The listing builds one solid part. Answer for the finished solid, in the listing's coordinates (mm). A direction names the side the tool comes from. Give positions to 0.01 mm unless a question says otherwise; leave off trailing zeros. Write each loop counter-clockwise with the first axis right and the second up, starting at its lowest first coordinate (ties: lowest second). Pieces come first, ordered by that corner, then holes. Notation, with made-up numbers: (60.5, 1) - (91.5, 1) arc R16 ccw to (91.5, 21) - close; hole circle Ø9 at (61.5, 62). An arc over 180 degrees is marked (long way). Answer as CSV lines item,"result". Start each with the question number.
(1) Find section A-A (x = 0). Write down the section's boundary in (y, z), then the cut area to 3 significant figures.
(2) Find section B-B (z = 9). Write down the section's boundary in (x, y), then the cut area to 3 significant figures.
(3) For faces 1 (the face through (15.294, 0, 5)), 2 (the face through (-9.228, -3.186, 2.465)), 3 (the face through (0, -4.7, 8)), determine the directions among +Z, -Z, +X, -X, +Y, -Y from which every point of the face is accessible in a straight line to the end or side of a thin tool.
(4) Find section C-C (z = 3.5). State how many separate pieces and enclosed holes the cut face has, then the cut area to 3 significant figures.
(5) Each of these flat-tipped pins is pushed along its axis until it touches: pin 1 Ø7 at (x, y) = (1.5, 2) entering from -Z; pin 2 Ø3 at (x, y) = (-11, -1.5) entering from -Z. Where does it stop, or does it pass through?
(6) Find section D-D (x = -7). Write down the section's boundary in (y, z), then the cut area to 3 significant figures.
(7) For a pull along X with two mould halves and no side action, classify faces 4 (the face through (0, -8, 0)), 5 (the face through (5.15, -1.77, 7.98)), 6 (the face through (-14.09, 7.44, 4.82)), 7 (the face through (14.154, -7.374, 4.816)) as pulls with the +X half, pulls with the -X half, needs draft (parallel to the pull), parting line crosses it, or undercut.
(8) Straight lines are drawn through the part: probe 1 along Y at (x, z) = (3, 1.5); probe 2 along X at (y, z) = (-1.5, 8.5); probe 3 along X at (y, z) = (4.25, 5.25). For each, find the intervals that lie inside material, in ascending order.
from build123d import *

# Parameters (mm, degrees)
SKETCH041_W     = 30.588764
SKETCH041_H     = 17.153068
PAD012_DEPTH    = 10
SKETCH042_W     = 18
SKETCH042_H     = 14
POCKET033_DEPTH = 6
POCKET034_DEPTH = 5
POCKET035_DEPTH = 10.001
SKETCH045_R     = 1.272634
PAD013_DEPTH    = 3
CHAMFER011_SIZE = 1
FILLET033_R     = 0.8
FILLET034_R     = 4
FILLET035_R     = 0.5


with BuildPart() as part:
    # Sketch041 → Pad012 (new body)
    with BuildSketch(Plane.XY):
        Rectangle(SKETCH041_W, SKETCH041_H)
    extrude(amount=PAD012_DEPTH)

    # Sketch042 → Pocket033 (cut)
    with BuildSketch(Plane.XY):
        Rectangle(SKETCH042_W, SKETCH042_H)
    extrude(amount=POCKET033_DEPTH, mode=Mode.SUBTRACT)

    # Sketch043 → Pocket034 (cut)
    with BuildSketch(Plane.XY):
        with BuildLine():
            ThreePointArc((-9.861316, 2.945018), (-12.806334, 0), (-9.861316, -2.945018))
            Line((-9.861316, -2.945018), (9.861316, -2.945018))
            ThreePointArc((9.861316, -2.945018), (12.806334, 0), (9.861316, 2.945018))
            Line((9.861316, 2.945018), (-9.861316, 2.945018))
        make_face()
    extrude(amount=POCKET034_DEPTH, mode=Mode.SUBTRACT)

    # Sketch044 → Pocket035 (cut, through all)
    with BuildSketch(Plane.XY):
        with BuildLine():
            ThreePointArc((-2.15, 1.3), (-5.15, -1.7), (-2.15, -4.7))
            Line((-2.15, -4.7), (2.15, -4.7))
            ThreePointArc((2.15, -4.7), (5.15, -1.7), (2.15, 1.3))
            Line((2.15, 1.3), (-2.15, 1.3))
        make_face()
    extrude(amount=POCKET035_DEPTH, mode=Mode.SUBTRACT)

    # Sketch045 (on Face21 of Pocket035) → Pad013 (join)
    with BuildSketch(Plane(origin=(0, 0, 6), x_dir=(1, 0, 0), z_dir=(0, 0, -1))):
        with Locations((-9.839489, 0)):
            Circle(SKETCH045_R)
        with Locations((9.839489, 0)):
            Circle(SKETCH045_R)
    extrude(amount=PAD013_DEPTH)

    # Chamfer011
    chamfer011_edges = [part.edges().sort_by_distance(p)[0] for p in [
        (8.566855, 0, 3),
        (-11.112123, 0, 3),
    ]]
    chamfer(chamfer011_edges, length=CHAMFER011_SIZE)

    # Fillet033
    fillet033_edges = [part.edges().sort_by_distance(p)[0] for p in [
        (9, 2.945018, 2.5),
        (9, -2.945018, 2.5),
        (9, 7, 3),
        (-9, 2.945018, 2.5),
        (-9, -2.945018, 2.5),
        (-9, -7, 3),
        (9, -7, 3),
        (-9, 7, 3),
    ]]
    fillet(fillet033_edges, radius=FILLET033_R)

    # Fillet034
    fillet034_edges = [part.edges().sort_by_distance(p)[0] for p in [
        (-15.294382, -8.576534, 5),
        (-15.294382, 8.576534, 5),
        (15.294382, 8.576534, 5),
        (15.294382, -8.576534, 5),
    ]]
    fillet(fillet034_edges, radius=FILLET034_R)

    # Fillet035
    fillet035_edges = [part.edges().sort_by_distance(p)[0] for p in [
        (0, 8.576534, 10),
        (-14.12281, 7.404962, 10),
        (14.12281, 7.404962, 10),
        (-15.294382, 0, 10),
        (15.294382, 0, 10),
        (-14.12281, -7.404962, 10),
        (14.12281, -7.404962, 10),
        (0, -8.576534, 10),
        (0, -4.7, 10),
        (5.15, -1.7, 10),
        (0, 1.3, 10),
        (-5.15, -1.7, 10),
        (-5.15, -1.7, 6),
    ]]
    fillet(fillet035_edges, radius=FILLET035_R)


solid = part.part
Result set:
1,outline,"(-8.58, 0) - (-7, 0) - (-7, 6) - (-5.2, 6) arc R0.5 ccw to (-4.7, 6.5) - (-4.7, 9.5) arc R0.5 ccw to (-5.2, 10) - (-8.08, 10) arc R0.5 ccw to (-8.58, 9.5) - close; (1.3, 6.5) arc R0.5 ccw to (1.8, 6) - (7, 6) - (7, 0) - (8.58, 0) - (8.58, 9.5) arc R0.5 ccw to (8.08, 10) - (1.8, 10) arc R0.5 ccw to (1.3, 9.5) - close"
1,area,"63.2 mm^2"
2,outline,"(-15.29, -4.58) arc R4 ccw to (-11.29, -8.58) - (11.29, -8.58) arc R4 ccw to (15.29, -4.58) - (15.29, 4.58) arc R4 ccw to (11.29, 8.58) - (-11.29, 8.58) arc R4 ccw to (-15.29, 4.58) - close; hole (-2.15, -4.7) - (2.15, -4.7) arc R3 ccw to (2.15, 1.3) - (-2.15, 1.3) arc R3 ccw to start"
2,area,"457 mm^2"
3,face 1,"+Z, -Z, +X, +Y, -Y"
3,face 2,"-Z"
3,face 3,"+Z, -Z"
4,separate pieces,"3"
4,enclosed holes,"1"
4,area,"225 mm^2"
5,pin 1,"z = 6"
5,pin 2,"z = 0"
6,outline,"(-8.58, 0) - (-7, 0) - (-7, 6) - (7, 6) - (7, 0) - (8.58, 0) - (8.58, 9.5) arc R0.5 ccw to (8.08, 10) - (-8.08, 10) arc R0.5 ccw to (-8.58, 9.5) - close"
6,area,"87.4 mm^2"
7,face 4,"needs draft"
7,face 5,"undercut"
7,face 6,"pulls with the -X half"
7,face 7,"pulls with the +X half"
8,probe 1,"-8.58 to -7, 7 to 8.58"
8,probe 2,"-15.29 to -5.14, 5.14 to 15.29"
8,probe 3,"-15.29 to -9, 9 to 15.29"
